The drawing under review shows one solid part. Ordinate dimensions are in mm from its lowest x, y, z. A direction names the side the tool comes from. Give positions to 0.01 mm unless a question says otherwise; leave off trailing zeros. Loops run counter-clockwise (first coordinate to the right, second up) from the corner with the lowest first, then second, coordinate; pieces in that order, holes last. Notation, with made-up numbers: M 11.25,80 L 52.25,80 A23 ccw 52.25,108 Z; hole C 77.5,-39 d6. An arc over 180 degrees is marked long. Write item = value, one per line. Start each with the question number.
1. We need section A-A on x = 0.3. Give the boundary of the cut face in (y, z).
2. We need section D-D on x = 1.5. Give the boundary of the cut face in (y, z).
3. We need section C-C on y = 5.75. Give the boundary of the cut face in (x, z).
4. We need section B-B on z = 6.5. Give the boundary of the cut face in (x, y).
5. For the marked faces 1, 2, 3 and 4, list the 3-axis set-ups (+Z, -Z, +X, -X, +Y, -Y) from which the entire face can be reached by the end or side of a thin tool; tool diameter is ignored.
6. Wall thickness on line 1 along Y through (x, z) = (1, 5.75); line 2 along Y through (x, z) = (1.2, 13.5); line 3 along Z through (x, y) = (2.6, 10): over which ranges is each line inside the solid? List them lowest first. Write a range as from..to.
7. For pin 1 (0.9 mm diameter, centred on x = 2, z = 6.5, fed in from +Y); pin 2 (1.5 mm diameter, centred on x = 1.5, y = 10, fed in from +Z), all flat-tipped, find the tip position at first contact; note any pin that passes through.
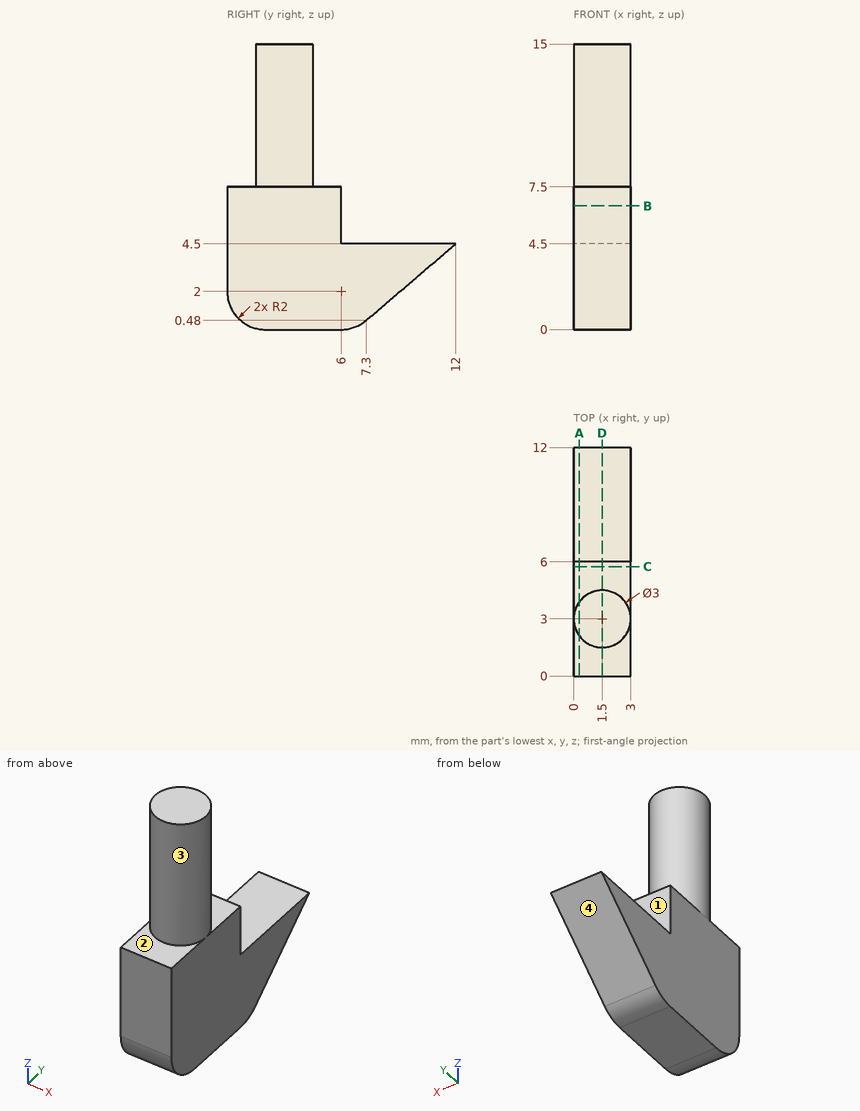
Final values:
q1.outline = M 0,2 A2 ccw 2,0 L 6,0 A2 ccw 7.3,0.48 L 12,4.5 L 6,4.5 L 6,7.5 L 3.9,7.5 L 3.9,15 L 2.1,15 L 2.1,7.5 L 0,7.5 Z
q2.outline = M 0,2 A2 ccw 2,0 L 6,0 A2 ccw 7.3,0.48 L 12,4.5 L 6,4.5 L 6,7.5 L 4.5,7.5 L 4.5,15 L 1.5,15 L 1.5,7.5 L 0,7.5 Z
q3.outline = M 0,0 L 3,0 L 3,7.5 L 0,7.5 Z
q4.outline = M 0,0 L 3,0 L 3,6 L 0,6 Z
q5.face_1 = +Z, +X, -X, +Y
q5.face_2 = +Z, -Y
q5.face_3 = +Z
q5.face_4 = -Z, +X, -X, +Y
q6.line_1 = 0..6
q6.line_2 = 1.53..4.47
q6.line_3 = 2.79..4.5
q7.pin_1 = 6
q7.pin_2 = 4.5
